from build123d import *

# Parameters (mm, degrees)
SKETCH1_W           = 1950
SKETCH1_H           = 1950
BOSS_EXTRUDE1_DEPTH = 2.4
SKETCH2_R           = 91.2
SKETCH2_R_2         = 35.65
SKETCH2_R_3         = 65.8
CUT_EXTRUDE1_DEPTH  = 3.4


with BuildPart() as part:
    # Sketch1 → Boss-Extrude1 (new body)
    with BuildSketch(Plane.XY):
        Rectangle(SKETCH1_W, SKETCH1_H)
    extrude(amount=BOSS_EXTRUDE1_DEPTH)

    # Sketch2 → Cut-Extrude1 (cut, through all)
    with BuildSketch(Plane.XY.offset(2.4)):
        Circle(SKETCH2_R)
        with Locations((0, 140)):
            Circle(SKETCH2_R_2)
        with Locations((222, 382)):
            Circle(SKETCH2_R)
        with Locations((-222, -382)):
            Circle(SKETCH2_R)
        with Locations((-900, 900)):
            Circle(SKETCH2_R_3)
        with Locations((-900, -900)):
            Circle(SKETCH2_R_3)
        with Locations((0, -140)):
            Circle(SKETCH2_R_2)
        with Locations((900, 900)):
            Circle(SKETCH2_R_3)
        with Locations((140, 0)):
            Circle(SKETCH2_R_2)
        with Locations((-140, 0)):
            Circle(SKETCH2_R_2)
        with Locations((900, -900)):
            Circle(SKETCH2_R_3)
    extrude(amount=-CUT_EXTRUDE1_DEPTH, mode=Mode.SUBTRACT)


solid = part.part
Can you work these out from the model? Positions are in its coordinate system, mm. Coordinates: 2 decimals unless noted, no trailing zeros. Write each loop counter-clockwise with the first axis right and the second up, starting at its lowest first coordinate (ties: lowest second). Pieces come first, ordered by that corner, then holes.
Q1. Imagine slicing it at C-C, the plane x = 900. List the corners of the cut face in (y, z) for me, plus the area to 3 significant figures.
Results found:
outline: (-975, 0) - (-965.8, 0) - (-965.8, 2.4) - (-975, 2.4) - close; (-834.2, 0) - (834.2, 0) - (834.2, 2.4) - (-834.2, 2.4) - close; (965.8, 0) - (975, 0) - (975, 2.4) - (965.8, 2.4) - close
area: 4,050 mm2
Q2. Please list where these lines run through material, in increasing order: L1, parallel to Y at x = 900, z = 0.75; L2, parallel to Y at x = 0, z = 0.7; L3, parallel to Y at x = -140, z = 1.85.
Results found:
L1: y = -975 to -965.8, -834.2 to 834.2, 965.8 to 975
L2: y = -975 to -175.65, -104.35 to -91.2, 91.2 to 104.35, 175.65 to 975
L3: y = -975 to -421.92, -342.08 to -35.65, 35.65 to 975
Q3. Imagine slicing it at A-A, the plane y = 140. List the corners of the cut face in (x, z) for me.
Results found:
outline: (-975, 0) - (-35.65, 0) - (-35.65, 2.4) - (-975, 2.4) - close; (35.65, 0) - (975, 0) - (975, 2.4) - (35.65, 2.4) - close
Q4. If we mould it in two halves opening along Y, with no side actions, what happens to faces 1 (the face through (203, 14, 2.4)), 2 (the face through (210.128, 472.424, 1.217)), 3 (the face through (-233.872, -291.576, 1.217))? For each: +Y half, -Y half, draft (parallel to the pull), parting line (faces both ways), or undercut.
Results found:
face 1: draft
face 2: undercut
face 3: undercut
Q5. Imagine slicing it at B-B, the plane z = 1.8. Count the separate pieces of the cut face and the enclosed holes in it, plus the area to 3 significant figures.
Results found:
separate pieces: 1
enclosed holes: 11
area: 3,650,000 mm2
